The listing builds one solid part. Answer for the finished solid, in the listing's coordinates (mm). A direction names the side the tool comes from. Round coordinates to 2 decimals unless told otherwise and drop trailing zeros. Write each loop counter-clockwise with the first axis right and the second up, starting at its lowest first coordinate (ties: lowest second). Pieces come first, ordered by that corner, then holes. Notation, with made-up numbers: (26.5, 35) - (31.5, 35) arc R29 cw to (31.5, 63) - close; hole circle Ø3 at (70, -15.75). An arc over 180 degrees is marked (long way). Answer in a Markdown table with one row per item.
from build123d import *
from build123d.topology import SkipClean

# Parameters (mm, degrees)
SALIENTE_EXTRUIR1_DEPTH    = 4.5
CORTAR_EXTRUIR4_DEPTH      = 10
CORTAR_EXTRUIR4_DEPTH_BACK = 28.546551508
CROQUIS7_R                 = 0.875
CORTAR_EXTRUIR5_DEPTH      = 11
CROQUIS9_R                 = 1.125
CORTAR_EXTRUIR6_DEPTH      = 27.234519245


with BuildPart() as part:
    # Croquis1 → Saliente-Extruir1 (new body)
    with BuildSketch(Plane(origin=(0, 0, 0), x_dir=(1, 0, 0), z_dir=(0, 1, 0))):
        with BuildLine():
            Line((-5, -10), (5, -10))
            Line((5, -10), (5, 10))
            Line((5, 10), (-5, 10))
            ThreePointArc((-5, 10), (-7.121320344, 9.121320344), (-8, 7))
            Line((-8, 7), (-8, 5.703831235))
            ThreePointArc((-8, 5.703831235), (-8.865157138, 3.615157138), (-10.953831235, 2.75))
            Line((-10.953831235, 2.75), (-24, 2.75))
            Line((-24, 2.75), (-24, 0.75))
            Line((-24, 0.75), (-8, 0.75))
            Line((-8, 0.75), (-8, -0.75))
            Line((-8, -0.75), (-24, -0.75))
            Line((-24, -0.75), (-24, -2.75))
            Line((-24, -2.75), (-10.953831235, -2.75))
            ThreePointArc((-10.953831235, -2.75), (-8.865157138, -3.615157138), (-8, -5.703831235))
            Line((-8, -5.703831235), (-8, -7))
            ThreePointArc((-8, -7), (-7.121320344, -9.121320344), (-5, -10))
        make_face()
    extrude(amount=SALIENTE_EXTRUIR1_DEPTH)

    # Croquis7 → Cortar-Extruir4 (cut, two sides: drawn at the far end of the back side and taken through both)
    with BuildSketch(Plane.XY.offset(2.75).offset(-CORTAR_EXTRUIR4_DEPTH_BACK)):
        with Locations(Location((-22, 2.25, 0), (0, 0, 180))):
            Circle(CROQUIS7_R)
        with Locations(Location((-17.5, 2.25, 0), (0, 0, 180))):
            Circle(CROQUIS7_R)
    extrude(amount=CORTAR_EXTRUIR4_DEPTH + CORTAR_EXTRUIR4_DEPTH_BACK, mode=Mode.SUBTRACT)

    # Croquis8 → Cortar-Extruir5 (cut)
    with BuildSketch(Plane(origin=(5, 0, 0), x_dir=(0, 0, -1), z_dir=(1, 0, 0))):
        Polygon((-8, 1), (8, 1), (8, 3.5), (5.5, 3.5), (5.5, 4.5), (-5.5, 4.5), (-5.5, 3.5), (-8, 3.5), align=None)
    extrude(amount=-CORTAR_EXTRUIR5_DEPTH, mode=Mode.SUBTRACT)

    # Croquis9 → Cortar-Extruir6 (cut, through all)
    with BuildSketch(Plane(origin=(0, 1, 0), x_dir=(1, 0, 0), z_dir=(0, 1, 0))):
        with Locations(Location((-4, 0, 0), (0, 0, 270))):
            Circle(CROQUIS9_R)
    extrude(amount=-CORTAR_EXTRUIR6_DEPTH, mode=Mode.SUBTRACT)

    # Croquis11 → Revolución2 (revolve)
    with SkipClean():  # the faces are left unmerged after this step: merging them gives an invalid solid
        with BuildSketch(Plane(origin=(0, 0, 0), x_dir=(0, 0, -1), z_dir=(1, 0, 0))):
            with BuildLine():
                Line((-0.5, 1), (0.5, 1))
                ThreePointArc((0.5, 1), (0, 1.5), (-0.5, 1))
            make_face()
        revolve(axis=Axis((0, 1, 0.5), (0, 0, -1)))


solid = part.part
(1) Flat-ended cylindrical pins translate along their axes: pin 1 (2 mm diameter, centred on x = -17, y = 3.5, fed in from -Z); pin 2 (2.5 mm diameter, centred on x = -17.5, y = 2.25, fed in from +Z); pin 3 (0.6 mm diameter, centred on y = 2, z = -6, fed in from -X). Find the tip coordinate at first contact, or state that the pin passes through.
Checked values:
| item | result |
|---|---|
| pin 1 | stops at z = -2.75 |
| pin 2 | stops at z = 2.75 |
| pin 3 | stops at x = -8 |
(2) Section B-B (z = 0) is taken. Give the vertices of the cut face in (x, y) (3 decimals).
Checked values:
| item | result |
|---|---|
| outline | (-8, 0) - (-5.125, 0) - (-5.125, 1) - (-6, 1) - (-6, 4.5) - (-8, 4.5) - close; (-2.875, 0) - (5, 0) - (5, 1) - (0.5, 1) arc R0.5 ccw to (-0.5, 1) - (-2.875, 1) - close |
(3) Section C-C (x = -22) is taken. Give the vertices of the cut face in (y, z) (3 decimals).
Checked values:
| item | result |
|---|---|
| outline | (0, -2.75) - (1.375, -2.75) - (1.375, -0.75) - (0, -0.75) - close; (0, 0.75) - (1.375, 0.75) - (1.375, 2.75) - (0, 2.75) - close; (3.125, -2.75) - (4.5, -2.75) - (4.5, -0.75) - (3.125, -0.75) - close; (3.125, 0.75) - (4.5, 0.75) - (4.5, 2.75) - (3.125, 2.75) - close |
(4) For faces 5 (the flat face through (-17, 1, -2.75)), 6 (the flat face through (0, 2, -8)), 7 (the flat face through (-18, 1, 2.75)), determine the directions among +Z, -Z, +X, -X, +Y, -Y from which every point of the face is accessible in a straight line to the end or side of a thin tool.
Checked values:
| item | result |
|---|---|
| face 5 | -Z, -X, +Y, -Y |
| face 6 | +X |
| face 7 | +Z, -X, +Y, -Y |
(5) For a pull along Z with two mould halves and no side action, classify faces 1 (the flat face through (0, 4, 5.5)), 2 (the flat face through (-16, 2, 0.75)), 3 (the cylindrical face through (-8.89, 2.22, 3.59)), 4 (the cylindrical face through (-7.1, 2.22, -9.14)) as pulls with the +Z half, pulls with the -Z half, needs draft (parallel to the pull), parting line crosses it, or undercut.
Checked values:
| item | result |
|---|---|
| face 1 | undercut |
| face 2 | undercut |
| face 3 | pulls with the +Z half |
| face 4 | pulls with the -Z half |
(6) Find the intervals of material crossed by line 1 (X direction, y = 2.3, z = 1.75); line 2 (Z direction, x = -2.5, y = 2.8); line 3 (Y direction, x = -17.5, z = -2.25) (3 decimals), in increasing order.
Checked values:
| item | result |
|---|---|
| line 1 | x = -24 to -22.87, -21.13 to -18.37, -16.63 to -6 |
| line 2 | z = -10 to -8, 8 to 10 |
| line 3 | y = 0 to 1.375, 3.125 to 4.5 |
(7) Section A-A (x = -13.5) is taken. Give the vertices of the cut face in (y, z), and give its area (3 significant figures).
Checked values:
| item | result |
|---|---|
| outline | (0, -2.75) - (4.5, -2.75) - (4.5, -0.75) - (0, -0.75) - close; (0, 0.75) - (4.5, 0.75) - (4.5, 2.75) - (0, 2.75) - close |
| area | 18.0 mm2 |
(8) Section D-D (z = 6.25) is taken. Give the vertices of the cut face in (x, y), and give its area (3 significant figures).
Checked values:
| item | result |
|---|---|
| outline | (-8, 0) - (5, 0) - (5, 1) - (-6, 1) - (-6, 3.5) - (5, 3.5) - (5, 4.5) - (-8, 4.5) - close |
| area | 31.0 mm2 |
